CAD build for the part. Positions are in the model's coordinates, mm. A direction names the side the tool comes from. Give positions to 0.01 mm unless a question says otherwise; leave off trailing zeros. Loops run counter-clockwise (first coordinate to the right, second up) from the corner with the lowest first, then second, coordinate; pieces in that order, holes last.
Item 1: Saw through at D-D on y = -2.75. Give the cut face in (x, z) (1 decimal).
Item 2: Which spindle directions (+Z, -Z, +X, -X, +Y, -Y) get a long thin tool onto all of the face, cutting with end or side? Do faces 1 (the flat face through (-12, 4, 9.525)), 2 (the cylindrical face through (12.95, 1.97, 10.31)), 3 (the flat face through (4, 4, 11.112)). Say none if no direction does.
Item 3: Saw through at C-C on z = 8.75. Give the cut face in (x, y) (1 decimal).
Item 4: Mould opens along X. For faces 4 (the flat face through (-15.875, 2, 5)), 5 (the flat face through (0, 3, 7.938)), 6 (the flat face through (0, 7, 0)) say: released by +X, released by -X, zero draft, split by the parting line, or undercut.
Item 5: Probe probe 1 along X at (y, z) = (2.25, 2.5) (1 decimal); probe 2 along X at (y, z) = (4.25, 10.5); probe 3 along Y at (x, z) = (13, 1.75). List the from-to ranges inside material, lowest first.
Item 6: Drop flat-ended pins along their axis: P1, Ø2, axis at x = -8.5, y = 4, coming from the +Z side (3 decimals); P2, Ø1.5, axis at x = 12, y = 4, coming from the -Z side; P3, Ø1.1, axis at x = -4, y = 4, coming from the -Z side (3 decimals); P4, Ø6, axis at y = -6, z = 10, coming from the -X side. Give the stop position or say it passes through.
from build123d import *

# Parameters (mm, degrees)
F0_W     = 31.75
F0_H     = 15.875
F0_R     = 2.2550277878
F1_DEPTH = 9.525
F2_DEPTH = 11.1125
F4_DEPTH = 31.751
F5_T     = -1.5875


# Not quite as in the source:
# - a feature names something its author has since deleted; it is built from what else it names


with BuildPart() as f1:
    # F0 (on Top) → F1 (new body)
    with BuildSketch(Plane.XY):
        Rectangle(F0_W, F0_H)
        with Locations((-11.90625, 3.96875)):
            Circle(F0_R, mode=Mode.SUBTRACT)
        with Locations((-3.96875, 3.96875)):
            Circle(F0_R, mode=Mode.SUBTRACT)
        with Locations((3.96875, 3.96875)):
            Circle(F0_R, mode=Mode.SUBTRACT)
        with Locations((11.90625, 3.96875)):
            Circle(F0_R, mode=Mode.SUBTRACT)
    extrude(amount=F1_DEPTH)

    # F0 (on Top) → F2 (join)
    with BuildSketch(Plane.XY):
        with Locations((-11.90625, 3.96875)):
            Circle(F0_R)
        with Locations((-3.96875, 3.96875)):
            Circle(F0_R)
        with Locations((3.96875, 3.96875)):
            Circle(F0_R)
        with Locations((11.90625, 3.96875)):
            Circle(F0_R)
    extrude(amount=F2_DEPTH)

    # F3 (on face) → F4 (cut, through all)
    with BuildSketch(Plane.YZ.offset(15.875)):
        Polygon((-7.9375, 9.525), (-7.9375, 3.175), (0, 9.525), align=None)
    extrude(amount=-F4_DEPTH, mode=Mode.SUBTRACT)

    # F5
    f5_openings = [f1.faces().sort_by_distance(p)[0] for p in [
        (0, 0, 0),
    ]]
    offset(amount=F5_T, openings=f5_openings, kind=Kind.INTERSECTION)


solid = f1.part
Results below:
1. outline: (-15.9, 0) - (-14.3, 0) - (-14.3, 5.3) - (14.3, 5.3) - (14.3, 0) - (15.9, 0) - (15.9, 7.3) - (-15.9, 7.3) - close
2. face 1: -Z
2. face 2: +Z
2. face 3: +Z, +X, -X, +Y, -Y
3. outline: (-15.9, -1) - (15.9, -1) - (15.9, 7.9) - (-15.9, 7.9) - close; hole circle Ø1.3 at (-11.9, 4); hole circle Ø1.3 at (-4, 4); hole circle Ø1.3 at (4, 4); hole circle Ø1.3 at (11.9, 4)
4. face 4: released by -X
4. face 5: undercut
4. face 6: zero draft
5. probe 1: x = -15.9 to -14.3, 14.3 to 15.9
5. probe 2: x = -14.14 to -9.67, -6.21 to -1.73, 1.73 to 6.21, 9.67 to 14.14
5. probe 3: y = -7.94 to -6.35, 6.35 to 7.94
6. P1: stops at z = 9.525
6. P2: stops at z = 7.94
6. P3: stops at z = 9.525
6. P4: passes through
